Check sheet for the modelled part. Datum: model origin and axes. Units: mm. Give positions to 0.01 mm unless a question says otherwise; leave off trailing zeros. Loops run counter-clockwise (first coordinate to the right, second up) from the corner with the lowest first, then second, coordinate; pieces in that order, holes last. Notation, with made-up numbers: (69, 62) - (118, 62) arc R17 cw to (118, 67) - close; hole circle Ø1 at (-2.75, 44.25). An arc over 180 degrees is marked (long way). Answer in a Markdown table with one row per item. Add a question column.
(1) Sectioned sample at C-C on y = 1.55. Enter the section's corners in (x, z).
(2) Draft check along X on faces 1 (the face through (-49.3, 1, -75.6)), 2 (the face through (-41.707, 1.014, -36.824)), 3 (the face through (-51, 0, -7)). Enter one of: released by +X, released by -X, zero draft, split by the parting line, or undercut.
(3) Go/stop test with flat-tipped pins: P1, Ø1, axis at x = -82, y = 1.5, coming from the +Z side; P2, Ø22.5, axis at x = -50.15, z = -27.61, coming from the -Y side. Record where each tip stops, or that it passes through.
(4) Thickness scan on L1, parallel to X at y = 1.2, z = -27; L2, parallel to X at y = 1.7, z = 5; L3, parallel to Z at x = -43, y = 0.65. Record the ranges inside material, lowest first.
(5) Sectioned sample at B-B on z = -17. Enter the section's corners in (x, y).
(6) Sectioned sample at A-A on x = -55.5. Enter the section's corners in (y, z).
(7) Sectioned sample at D-D on x = -35.5. Enter the section's corners in (y, z).
from build123d import *

# Parameters (mm, degrees)
BOSS_EXTRUDE1_DEPTH = 2
SKETCH2_R           = 12.5
SKETCH2_W           = 15
SKETCH2_H           = 50
CUT_EXTRUDE1_DEPTH  = 2


with BuildPart() as part:
    # Sketch1 → Boss-Extrude1 (new body)
    with BuildSketch(Plane(origin=(0, 0, 0), x_dir=(1, 0, 0), z_dir=(0, 1, 0))):
        with BuildLine():
            Line((-90.154867257, 35.610619469), (-90.154867257, -37.389380531))
            Line((-90.154867257, -37.389380531), (-10.154867257, -37.389380531))
            Line((-10.154867257, -37.389380531), (-10.154867257, 35.610619469))
            ThreePointArc((-10.154867257, 35.610619469), (-50.154867257, 75.610619469), (-90.154867257, 35.610619469))
        make_face()
    extrude(amount=BOSS_EXTRUDE1_DEPTH)

    # Sketch2 → Cut-Extrude1 (cut)
    with BuildSketch(Plane(origin=(0, 2, 0), x_dir=(1, 0, 0), z_dir=(0, 1, 0))):
        with Locations(Location((-50.154867257, 27.610619469, 0), (0, 0, 270))):
            Circle(SKETCH2_R)
        with Locations((-82.654867257, -12.389380531)):
            Rectangle(SKETCH2_W, SKETCH2_H)
        with Locations((-17.654867257, -12.389380531)):
            Rectangle(SKETCH2_W, SKETCH2_H)
    extrude(amount=-CUT_EXTRUDE1_DEPTH, mode=Mode.SUBTRACT)


solid = part.part
Reply:
| question | item | result |
|---|---|---|
| 1 | outline | (-90.15, -35.61) arc R40 ccw to (-10.15, -35.61) - (-10.15, -12.61) - (-25.15, -12.61) - (-25.15, 37.39) - (-75.15, 37.39) - (-75.15, -12.61) - (-90.15, -12.61) - close; hole circle Ø25 at (-50.15, -27.61) |
| 2 | face 1 | split by the parting line |
| 2 | face 2 | undercut |
| 2 | face 3 | zero draft |
| 3 | P1 | z = -12.61 |
| 3 | P2 | through |
| 4 | L1 | -90.15 to -62.64, -37.67 to -10.15 |
| 4 | L2 | -75.15 to -25.15 |
| 4 | L3 | -74.97 to -37.86, -17.36 to 37.39 |
| 5 | outline | (-90.15, 0) - (-56.76, 0) - (-56.76, 2) - (-90.15, 2) - close; (-43.55, 0) - (-10.15, 0) - (-10.15, 2) - (-43.55, 2) - close |
| 6 | outline | (0, -75.25) - (2, -75.25) - (2, -38.91) - (0, -38.91) - close; (0, -16.31) - (2, -16.31) - (2, 37.39) - (0, 37.39) - close |
| 7 | outline | (0, -72.83) - (2, -72.83) - (2, 37.39) - (0, 37.39) - close |
